Input: part model. Units: mm. Frame: model coordinates. A direction names the side the tool comes from. Round coordinates to 2 decimals unless told otherwise and drop trailing zeros. Write each loop counter-clockwise with the first axis right and the second up, starting at its lowest first coordinate (ties: lowest second). Pieces come first, ordered by that corner, then holes. Notation, with made-up numbers: (-7, -35.5) -> (32, -35.5) arc R7 ccw to (32, -30.5) -> close; hole circle Ø2 at (-7, 39). An arc over 180 degrees is marked (long way). Write item = value, one per line. Start each with the question number.
```python
from build123d import *

# Parameters (mm, degrees)
F0_W     = 460
F0_H     = 300
F1_DEPTH = 6
F2_W     = 460
F2_H     = 300
F2_W_2   = 448
F2_H_2   = 288
F3_DEPTH = 90
F4_R     = 4
F5_DEPTH = 460


with BuildPart() as f1:
    # F0 (on Top) → F1 (new body)
    with BuildSketch(Plane.XY):
        Rectangle(F0_W, F0_H)
    extrude(amount=F1_DEPTH)

    # F2 (on face) → F3 (join)
    with BuildSketch(Plane.XY.offset(6)):
        Rectangle(F2_W, F2_H)
        Rectangle(F2_W_2, F2_H_2, mode=Mode.SUBTRACT)
    extrude(amount=F3_DEPTH)

    # F4 (on face) → F5 (cut, through all)
    with BuildSketch(Plane(origin=(-230, 0, 0), x_dir=(0, -1, 0), z_dir=(-1, 0, 0))):
        with Locations((-120, 30)):
            Circle(F4_R)
        with Locations((120, 66)):
            Circle(F4_R)
    extrude(amount=-F5_DEPTH, mode=Mode.SUBTRACT)


solid = f1.part
```
1. Reachability of faces 1 (the flat face through (-3, 2, 6)), 2 (the flat face through (-1, 145, 96)) from +Z, -Z, +X, -X, +Y, -Y: full face, straight path, thin tool, end or side. Return the list, or none.
2. Section B-B (z = 80.5). Output: boundary loops of the cut face in (x, y).
3. Section A-A (y = 109). Output: boundary loops of the cut face in (x, z).
4. Section C-C (x = 149). Output: boundary loops of the cut face in (y, z).
5. Line query: line 1 along Y through (x, z) = (-172.5, 33); line 2 along Z through (x, y) = (225, -120); line 3 along X through (y, z) = (97.5, 19). Output: solid intervals per line, ascending.
6. Mould query, pull axis Y, two halves, no side actions, for faces 3 (the flat face through (230, -2, 47)), 4 (the flat face through (-3, 144, 50)), 5 (the flat face through (-3, -150, 47)). Classes: pulls with the +Y half, pulls with the -Y half, needs draft (parallel to the pull), parting line crosses it, or undercut.
7. Pin query (flat end, axial travel): P1, Ø1.5, axis at x = -183, y = -94.5, coming from the +Z side. Return the tip coordinate at first contact, or that it passes through.
Check sheet entries:
q1.face_1 = +Z
q1.face_2 = +Z, +X, -X, +Y, -Y
q2.outline = (-230, -150) -> (230, -150) -> (230, 150) -> (-230, 150) -> close; hole (-224, -144) -> (224, -144) -> (224, 144) -> (-224, 144) -> close
q3.outline = (-230, 0) -> (230, 0) -> (230, 96) -> (224, 96) -> (224, 6) -> (-224, 6) -> (-224, 96) -> (-230, 96) -> close
q4.outline = (-150, 0) -> (150, 0) -> (150, 96) -> (144, 96) -> (144, 6) -> (-144, 6) -> (-144, 96) -> (-150, 96) -> close
q5.line_1 = -150 to -144, 144 to 150
q5.line_2 = 0 to 62, 70 to 96
q5.line_3 = -230 to -224, 224 to 230
q6.face_3 = needs draft
q6.face_4 = undercut
q6.face_5 = pulls with the -Y half
q7.P1 = 6
